The model under review builds one solid part; all positions refer to its coordinate system, in mm. A direction names the side the tool comes from. Give positions to 0.01 mm unless a question says otherwise; leave off trailing zeros. Loops run counter-clockwise (first coordinate to the right, second up) from the corner with the lowest first, then second, coordinate; pieces in that order, holes last. Notation, with made-up numbers: M 56.5,-38.75 L 97.5,-38.75 A21 ccw 97.5,-11.75 Z; hole C -1.5,-7.5 d10. An arc over 180 degrees is marked long. One line per item, written item: value. Start each with the question number.
Q1. For faces 4 (the face through (19, 5, 34.925)), 5 (the face through (92.01, 4.83, 1.72)), 6 (the face through (6.35, 5, 27)), 7 (the face through (68, 5, -20)), 8 (the face through (86.93, 1.57, -10.7)), list the 3-axis set-ups (+Z, -Z, +X, -X, +Y, -Y) from which the entire face can be reached by the end or side of a thin tool; tool diameter is ignored.
Q2. For pin 1 (2 mm diameter, centred on x = 47.5, y = 2.5, fed in from -Z); pin 2 (5 mm diameter, centred on y = 5.5, z = 31, fed in from -X); pin 3 (11 mm diameter, centred on x = 98, z = -9.5, fed in from -Y) (3 decimals), all flat-tipped, find the tip position at first contact; note any pin that passes through.
Q3. Mouldability with a two-part tool opening along Z and no side actions: class faces 1 (the face through (58, 0, 14)), 2 (the face through (52.436, 4.696, -4.292)), 3 (the face through (24.636, 4.829, 10.249)) as released by +Z, released by -Z, zero draft, split by the parting line, or undercut.
Q4. To check wall thickness, follow line 1 along Z through (x, y) = (17.5, 8.5) (3 decimals); line 2 along X through (y, z) = (1.6, 19.05); line 3 along X through (y, z) = (8.5, 18). State the ranges of each line that lie inside material, in increasing order. Write a range as from..to.
Q5. We need section D-D on z = 28.55. Write out the cut boundary in (x, y) (3 decimals).
Q6. We need section B-B on x = 20.5. Write out the cut boundary in (y, z) (3 decimals), plus the area to 3 significant figures.
Q7. We need section A-A on z = 19.05. Write out the cut boundary in (x, y) (3 decimals), plus the area to 3 significant figures.
Q8. We need section C-C on y = 1.75. Give the number of separate pieces and of enclosed holes in the cut face, plus the area to 3 significant figures.
```python
from build123d import *

# Parameters (mm, degrees)
SKETCH1_R           = 4.7625
SKETCH1_R_2         = 1.5
SKETCH1_R_3         = 3.175
BOSS_EXTRUDE1_DEPTH = 9.525
FILLET1_R           = 3.175
FILLET2_R           = 3.175
SKETCH2_R           = 14.5
CUT_EXTRUDE1_DEPTH  = 5.525
SKETCH3_R           = 12.7
CUT_EXTRUDE2_DEPTH  = 3.175
SKETCH4_W           = 12.7
SKETCH4_H           = 25.4
CUT_EXTRUDE3_DEPTH  = 10.525
FILLET3_R           = 2.54


with BuildPart() as part:
    # Sketch1 → Boss-Extrude1 (new body)
    with BuildSketch(Plane(origin=(0, 0, 0), x_dir=(1, 0, 0), z_dir=(0, 1, 0))):
        with BuildLine():
            Line((0, 0), (38.1, 0))
            ThreePointArc((38.1, 0), (52.620300687, 4.403064286), (63.218539249, 15.261399634))
            ThreePointArc((63.218539249, 15.261399634), (67.86863694, 19.924564568), (74.228922018, 21.631986448))
            Line((74.228922018, 21.631986448), (99.628922018, 21.631986448))
            ThreePointArc((99.628922018, 21.631986448), (110.444915242, 10.815993224), (99.628922018, 0))
            Line((99.628922018, 0), (88.9, 0))
            Line((88.9, 0), (114.3, -38.1))
            Line((114.3, -38.1), (6.35, -38.1))
            Line((6.35, -38.1), (6.35, -12.7))
            Line((6.35, -12.7), (0, -12.7))
            Line((0, -12.7), (0, 0))
        make_face()
        with Locations((99.628922018, 10.815993224)):
            Circle(SKETCH1_R, mode=Mode.SUBTRACT)
        with Locations((69.568539249, 15.261399634)):
            Circle(SKETCH1_R_2, mode=Mode.SUBTRACT)
        with Locations((82.268539249, 15.261399634)):
            Circle(SKETCH1_R_2, mode=Mode.SUBTRACT)
        with Locations((69.720479044, -19.05)):
            Circle(SKETCH1_R_2, mode=Mode.SUBTRACT)
        with Locations((61.720479044, -28.55)):
            Circle(SKETCH1_R_2, mode=Mode.SUBTRACT)
        with Locations((53.720479044, -19.05)):
            Circle(SKETCH1_R_2, mode=Mode.SUBTRACT)
        with Locations((61.720479044, -9.55)):
            Circle(SKETCH1_R_2, mode=Mode.SUBTRACT)
        with Locations((61.720479044, -19.05)):
            Circle(SKETCH1_R_3, mode=Mode.SUBTRACT)
    extrude(amount=BOSS_EXTRUDE1_DEPTH)

    # Fillet1
    fillet1_edges = [part.edges().sort_by_distance(p)[0] for p in [
        (88.9, 4.7625, 0),
    ]]
    fillet(fillet1_edges, radius=FILLET1_R)

    # Fillet2
    fillet2_edges = [part.edges().sort_by_distance(p)[0] for p in [
        (6.35, 4.7625, 12.7),
    ]]
    fillet(fillet2_edges, radius=FILLET2_R)

    # Sketch2 → Cut-Extrude1 (cut)
    with BuildSketch(Plane(origin=(0, 9.525, 0), x_dir=(1, 0, 0), z_dir=(0, 1, 0))):
        with Locations((61.720479044, -19.05)):
            Circle(SKETCH2_R)
    extrude(amount=-CUT_EXTRUDE1_DEPTH, mode=Mode.SUBTRACT)

    # Sketch3 → Cut-Extrude2 (cut)
    with BuildSketch(Plane(origin=(0, 0, 0), x_dir=(1, 0, 0), z_dir=(0, 1, 0))):
        with Locations((99.628922018, 10.815993224)):
            Circle(SKETCH3_R)
    extrude(amount=CUT_EXTRUDE2_DEPTH, mode=Mode.SUBTRACT)

    # Sketch4 → Cut-Extrude3 (cut, through all)
    with BuildSketch(Plane.XZ):
        with Locations((19.05, 22.225)):
            Rectangle(SKETCH4_W, SKETCH4_H)
    extrude(amount=-CUT_EXTRUDE3_DEPTH, mode=Mode.SUBTRACT)

    # Fillet3
    fillet3_edges = [part.edges().sort_by_distance(p)[0] for p in [
        (12.7, 4.7625, 34.925),
        (25.4, 4.7625, 34.925),
        (25.4, 4.7625, 9.525),
        (12.7, 4.7625, 9.525),
    ]]
    fillet(fillet3_edges, radius=FILLET3_R)


solid = part.part
```
Solved:
1. face 4: +Y, -Y
1. face 5: +X, +Y, -Y
1. face 6: +Z, -X, +Y, -Y
1. face 7: -Z, -X, +Y, -Y
1. face 8: +X, -Y
2. pin 1: z = -2.31
2. pin 2: x = 6.35
2. pin 3: y = 3.175
3. face 1: zero draft
3. face 2: released by -Z
3. face 3: undercut
4. line 1: 0..9.525, 34.925..38.1
4. line 2: 6.35..12.7, 25.4..52.22, 55.22..58.55, 64.9..68.22, 71.22..101.6
4. line 3: 6.35..12.7, 25.4..47.26, 76.18..100.9
5. outline: M 6.35,0 L 12.7,0 L 12.7,9.525 L 6.35,9.525 Z; M 25.4,0 L 60.22,0 L 60.22,4 L 50.766,4 L 50.766,9.525 L 25.4,9.525 Z; M 63.22,0 L 107.933,0 L 107.933,9.525 L 72.675,9.525 L 72.675,4 L 63.22,4 Z
6. outline: M 0,0 L 9.525,0 L 9.525,9.525 L 0,9.525 Z; M 0,34.925 L 9.525,34.925 L 9.525,38.1 L 0,38.1 Z
6. area: 121 mm2
7. outline: M 6.35,0 L 12.7,0 L 12.7,9.525 L 6.35,9.525 Z; M 25.4,0 L 52.22,0 L 52.22,4 L 47.22,4 L 47.22,9.525 L 25.4,9.525 Z; M 55.22,0 L 58.545,0 L 58.545,4 L 55.22,4 Z; M 64.895,0 L 68.22,0 L 68.22,4 L 64.895,4 Z; M 71.22,0 L 101.6,0 L 101.6,9.525 L 76.22,9.525 L 76.22,4 L 71.22,4 Z
7. area: 577 mm2
8. separate pieces: 1
8. enclosed holes: 8
8. area: 3,980 mm2
